```python
from build123d import *

# Parameters (mm, degrees)
CHAMFER_2_SIZE      = 1
CUT_EXTRUDE_1_DEPTH = 2


with BuildPart() as part:
    # 草图1 → 旋转1 (revolve)
    with BuildSketch(Plane.XY, mode=Mode.PRIVATE) as revolve_1_sk:
        Polygon((0, 0), (3, 0), (3, 8), (2, 8), (2, 10), (4.75, 10), (4.75, 18), (8, 18), (8, 22), (0, 22), align=None)
    revolve(revolve_1_sk.sketch.rotate(Axis((0, 22, 0), (0, -1, 0)), 180), axis=Axis((0, 22, 0), (0, -1, 0)))

    # 倒角2
    chamfer_2_edges = [part.edges().sort_by_distance(p)[0] for p in [
        (3, 8, 0),
        (3, 0, 0),
        (8, 22, 0),
    ]]
    chamfer(chamfer_2_edges, length=CHAMFER_2_SIZE - 0.0001)  # a hair under: the kernel refuses the full size

    # 草图2 → 切除-拉伸1 (cut)
    with BuildSketch(Plane(origin=(0, 22, 0), x_dir=(1, 0, 0), z_dir=(0, 1, 0))):
        with BuildLine():
            Line((-7.964766161, -0.75), (7.964766161, -0.75))
            ThreePointArc((7.964766161, -0.75), (8, 0), (7.964766161, 0.75))
            Line((7.964766161, 0.75), (-7.964766161, 0.75))
            ThreePointArc((-7.964766161, 0.75), (-8, 0), (-7.964766161, -0.75))
        make_face()
    extrude(amount=-CUT_EXTRUDE_1_DEPTH, mode=Mode.SUBTRACT)


solid = part.part
```
Can you work these out from the model? Positions are in its coordinate system, mm. A direction names the side the tool comes from. Coordinates: 2 decimals unless noted, no trailing zeros. Loops run counter-clockwise (first coordinate to the right, second up) from the corner with the lowest first, then second, coordinate; pieces in that order, holes last. Notation, with made-up numbers: (-18, 42.25) - (40, 42.25) arc R19 cw to (40, 60.25) - close; hole circle Ø10 at (-14, 36). An arc over 180 degrees is marked (long way). Use a Markdown table: item, result.
Item 1: For faces 1 (the face through (0, 21, 0.75)), 2 (the face through (-0.1, 21.8, -7.2)), 3 (the face through (0, 9, 2)), 4 (the face through (1.03, 14.056, 4.637)), 5 (the face through (-7.39, 19.52, 3.06)), which set-ups out of +Z, -Z, +X, -X, +Y, -Y let a thin tool reach every point of the face, with its end or its side?
Numbers:
| item | result |
|---|---|
| face 1 | +X, -X, +Y |
| face 2 | -Z, +Y |
| face 3 | none |
| face 4 | -Y |
| face 5 | +Y, -Y |
Item 2: I want a section at C-C on y = 13.5. Please give me the cut outline in (x, z).
Numbers:
| item | result |
|---|---|
| outline | circle Ø9.5 at (0, 0) |
Item 3: If I drill on probe 1 along Y at (x, z) = (6.75, -1.5); probe 2 along Z at (x, y) = (3.75, 20.75); probe 3 along Y at (x, z) = (4, -0.5), over which ranges is the centre line in solid material (lowest first)? Write a range as from..to.
Numbers:
| item | result |
|---|---|
| probe 1 | y = 18..22 |
| probe 2 | z = -7.07..-0.75, 0.75..7.07 |
| probe 3 | y = 10..20 |
Item 4: I want a section at D-D on y = 3.25. Please give me the cut outline in (x, z), and give its area (3 significant figures).
Numbers:
| item | result |
|---|---|
| outline | circle Ø6 at (0, 0) |
| area | 28.3 mm2 |
Item 5: We'd pull the mould along Y, two halves only. Please class faces 6 (the face through (2, 10, 1)), 7 (the face through (0, 21, -0.75)), 8 (the face through (0, 22, 3)): released by +Y, released by -Y, zero draft, split by the parting line, or undercut.
Numbers:
| item | result |
|---|---|
| face 6 | undercut |
| face 7 | zero draft |
| face 8 | released by +Y |
Item 6: Will these pins go through, and if not, where does the flat tip stop? pin 1 (3 mm diameter, centred on y = 13.5, z = -1.5, fed in from -X); pin 2 (5 mm diameter, centred on x = 4.5, y = 8.5, fed in from +Z); pin 3 (1 mm diameter, centred on x = 2.5, y = 6.5, fed in from -Z).
Numbers:
| item | result |
|---|---|
| pin 1 | stops at x = -4.75 |
| pin 2 | stops at z = 4.04 |
| pin 3 | stops at z = -2.24 |
